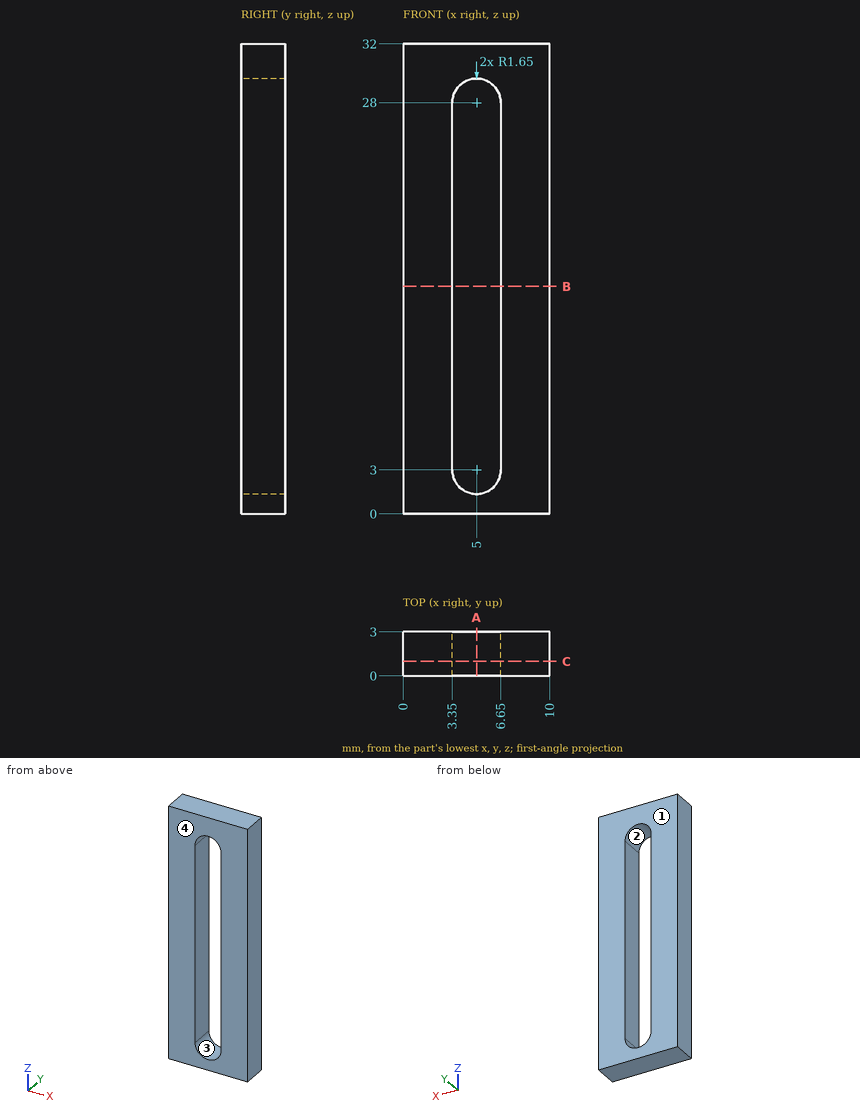
For this review, use the dimensioned drawing (mm, ordinates from the lowest corner) and the shaded views. A direction names the side the tool comes from. Give positions to 0.01 mm unless a question says otherwise; leave off trailing zeros. Loops run counter-clockwise (first coordinate to the right, second up) from the corner with the lowest first, then second, coordinate; pieces in that order, holes last. Notation, with made-up numbers: (63.5, 13) -> (83.5, 13) arc R25 cw to (83.5, 38) -> close; hole circle Ø2 at (88.5, 83.5). An arc over 180 degrees is marked (long way). One line per question, with ' | ' between items. Start each with the question number.
(1) For the marked faces 3 and 4, list the 3-axis set-ups (+Z, -Z, +X, -X, +Y, -Y) from which the entire face can be reached by the end or side of a thin tool; tool diameter is ignored.
(2) Draft analysis for pull direction Z (two halves, no side actions). For the marked faces 1 and 2, state which applies: +Z half, -Z half, draft (parallel to the pull), parting line (faces both ways), or undercut.
(3) We need section B-B (z = 15.5). State the section outline as (x, y) points, and give its area (3 significant figures).
(4) We need section C-C (y = 1). State the section outline as (x, z) points.
(5) We need section A-A (x = 5). State the section outline as (y, z) points.
(6) For line 1 (X direction, y = 0.7, z = 7); line 2 (X direction, y = 2.3, z = 29.5); line 3 (Z direction, x = 6, y = 1.2), list the stretches that pass through material, from the lowest coordinate up.
The answers:
1) face 3: +Y, -Y | face 4: +Z, -Z, +X, -X, -Y
2) face 1: draft | face 2: undercut
3) outline: (0, 0) -> (3.35, 0) -> (3.35, 3) -> (0, 3) -> close; (6.65, 0) -> (10, 0) -> (10, 3) -> (6.65, 3) -> close | area: 20.1 mm^2
4) outline: (0, 0) -> (10, 0) -> (10, 32) -> (0, 32) -> close; hole (3.35, 3) arc R1.65 ccw to (6.65, 3) -> (6.65, 28) arc R1.65 ccw to (3.35, 28) -> close
5) outline: (0, 0) -> (3, 0) -> (3, 1.35) -> (0, 1.35) -> close; (0, 29.65) -> (3, 29.65) -> (3, 32) -> (0, 32) -> close
6) line 1: x = 0 to 3.35, 6.65 to 10 | line 2: x = 0 to 4.31, 5.69 to 10 | line 3: z = 0 to 1.69, 29.31 to 32
